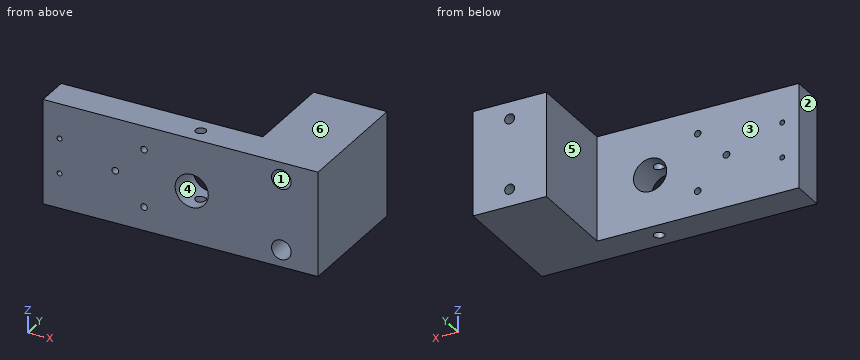
from build123d import *

# Parameters (mm, degrees)
SKETCH2_W                = 40
SKETCH2_H                = 12.7
BOSS_EXTRUDE1_DEPTH      = 105.35
SKETCH4_R                = 6.35
CUT_EXTRUDE1_DEPTH       = 13.7
F_4_0_4_DIAMETER_HOLE1_D = 4
SKETCH9_R                = 1.291519898
SKETCH9_R_2              = 1.25
CUT_EXTRUDE3_DEPTH       = 13.7000001
SKETCH14_W               = 28.1
SKETCH14_H               = 40
BOSS_EXTRUDE3_DEPTH      = 35.45
SKETCH10_R               = 3.75
CUT_EXTRUDE4_DEPTH       = 24.5
SKETCH15_R               = 1.905
CUT_EXTRUDE7_DEPTH       = 24.65
SKETCH17_R               = 0.95
CUT_EXTRUDE8_DEPTH       = 21


with BuildPart() as part:
    # Sketch2 → Boss-Extrude1 (new body)
    with BuildSketch(Plane(origin=(0, 0, 0), x_dir=(0, 0, -1), z_dir=(1, 0, 0))):
        with Locations((-8.031139822, -4.466363736)):
            Rectangle(SKETCH2_W, SKETCH2_H)
    extrude(amount=BOSS_EXTRUDE1_DEPTH)

    # Sketch4 → Cut-Extrude1 (cut, through all)
    with BuildSketch(Plane(origin=(0, 1.883636264, 0), x_dir=(1, 0, 0), z_dir=(0, 1, 0))):
        with Locations((56.96, -8.031139822)):
            Circle(SKETCH4_R)
    extrude(amount=-CUT_EXTRUDE1_DEPTH, mode=Mode.SUBTRACT)

    # Ø4.0 (4) Diameter Hole1 (through all)
    with Locations(Plane.XY.offset(28.031139822)):
        with Locations((56.96, -4.466363736)):
            Hole(F_4_0_4_DIAMETER_HOLE1_D / 2)

    # Sketch9 → Cut-Extrude3 (cut, through all)
    with BuildSketch(Plane(origin=(0, 1.883636264, 0), x_dir=(1, 0, 0), z_dir=(0, 1, 0))):
        with Locations((27.7, -8.031139822)):
            Circle(SKETCH9_R)
        with Locations((38.7, 2.968860178)):
            Circle(SKETCH9_R_2)
        with Locations((38.7, -19.031139822)):
            Circle(SKETCH9_R_2)
    extrude(amount=-CUT_EXTRUDE3_DEPTH, mode=Mode.SUBTRACT)

    # Sketch14 → Boss-Extrude3 (add)
    with BuildSketch(Plane(origin=(0, 1.883636264, 0), x_dir=(1, 0, 0), z_dir=(0, 1, 0))):
        with Locations((91.3, -8.031139822)):
            Rectangle(SKETCH14_W, SKETCH14_H)
    extrude(amount=BOSS_EXTRUDE3_DEPTH)

    # Sketch10 → Cut-Extrude4 (cut)
    with BuildSketch(Plane(origin=(0, -10.816363736, 0), x_dir=(1, 0, 0), z_dir=(0, 1, 0))):
        with Locations((91.3, -21.505839822)):
            Circle(SKETCH10_R)
        with Locations((91.3, 5.443560178)):
            Circle(SKETCH10_R)
    extrude(amount=CUT_EXTRUDE4_DEPTH, mode=Mode.SUBTRACT)

    # Sketch15 → Cut-Extrude7 (cut, through all)
    with BuildSketch(Plane.XZ.offset(-13.683636264)):
        with Locations((91.3, -5.443560178)):
            Circle(SKETCH15_R)
        with Locations((91.3, 21.505839822)):
            Circle(SKETCH15_R)
    extrude(amount=-CUT_EXTRUDE7_DEPTH, mode=Mode.SUBTRACT)

    # Sketch17 → Cut-Extrude8 (cut)
    with BuildSketch(Plane.XZ.offset(10.816363736)):
        with Locations((6.35, 14.698139822)):
            Circle(SKETCH17_R)
        with Locations((6.35, 1.364139822)):
            Circle(SKETCH17_R)
    extrude(amount=-CUT_EXTRUDE8_DEPTH, mode=Mode.SUBTRACT)


solid = part.part
Work out the finished part from the listing and answer in its coordinate system (mm). Face numbers are marked on the shaded views. A direction names the side the tool comes from. Coordinates: 2 decimals unless noted, no trailing zeros. Loops run counter-clockwise (first coordinate to the right, second up) from the corner with the lowest first, then second, coordinate; pieces in that order, holes last. Notation, with made-up numbers: M 65.25,50 L 89.25,50 A21 cw 89.25,65 Z; hole C 69,86.5 d9. An arc over 180 degrees is marked long. Answer in a Markdown table with one row per item. Add a question column.
1. The mould has two halves that part along X. Classify the marked faces 4, 5 and 6: pulls with the +X half, pulls with the -X half, needs draft (parallel to the pull), parting line crosses it, or undercut.
2. Find section B-B, the plane x = 27.7. Write down the section's boundary in (y, z).
3. Consider L1, parallel to Z at x = 38.7, y = -6.75; L2, parallel to Z at x = 56.96, y = -1; L3, parallel to Z at x = 90, y = -4. Determine where each line is inside the solid, lowest interval first.
4. Find section A-A, the plane x = 91.3. Write down the section's boundary in (y, z).
5. Flat-ended cylindrical pins translate along their axes: P1, Ø2, axis at y = 17, z = 0.5, coming from the -X side; P2, Ø8, axis at x = 89.5, z = -5, coming from the -Y side; P3, Ø4, axis at x = 38.7, z = 19.03, coming from the +Y side. Find the tip coordinate at first contact, or state that the pin passes through.
6. Find section C-C, the plane x = 56.96. Write down the section's boundary in (y, z), then the cut area to 3 significant figures.
7. A tool of negligible diameter and unlimited length cuts with its end or side. For the marked faces 1, 2 and 3, from which of +Z, -Z, +X, -X, +Y, -Y can it reach the whole face along a straight path? Write none if from no direction.
8. Find section D-D, the plane z = 3.5. Write down the section's boundary in (x, y), then the cut area to 3 significant figures.
Reported:
| question | item | result |
|---|---|---|
| 1 | face 4 | undercut |
| 1 | face 5 | pulls with the -X half |
| 1 | face 6 | needs draft |
| 2 | outline | M -10.82,-11.97 L 1.88,-11.97 L 1.88,6.74 L -10.82,6.74 Z; M -10.82,9.32 L 1.88,9.32 L 1.88,28.03 L -10.82,28.03 Z |
| 3 | L1 | z = -11.97 to -4.22, -1.72 to 17.78, 20.28 to 28.03 |
| 3 | L2 | z = -11.97 to 1.68, 14.38 to 28.03 |
| 3 | L3 | z = -11.97 to -8.96, -1.93 to 17.99, 25.02 to 28.03 |
| 4 | outline | M -10.82,-11.97 L 37.33,-11.97 L 37.33,-7.35 L 13.68,-7.35 L 13.68,-9.19 L -10.82,-9.19 Z; M -10.82,-1.69 L 13.68,-1.69 L 13.68,-3.54 L 37.33,-3.54 L 37.33,19.6 L 13.68,19.6 L 13.68,17.76 L -10.82,17.76 Z; M -10.82,25.26 L 13.68,25.26 L 13.68,23.41 L 37.33,23.41 L 37.33,28.03 L -10.82,28.03 Z |
| 5 | P1 | stops at x = 77.25 |
| 5 | P2 | stops at y = -10.82 |
| 5 | P3 | stops at y = 1.88 |
| 6 | outline | M -10.82,-11.97 L -6.47,-11.97 L -6.47,1.68 L -10.82,1.68 Z; M -10.82,14.38 L -6.47,14.38 L -6.47,28.03 L -10.82,28.03 Z; M -2.47,-11.97 L 1.88,-11.97 L 1.88,1.68 L -2.47,1.68 Z; M -2.47,14.38 L 1.88,14.38 L 1.88,28.03 L -2.47,28.03 Z |
| 6 | area | 238 mm^2 |
| 7 | face 1 | -Y |
| 7 | face 2 | +Z, -Z, -X, +Y, -Y |
| 7 | face 3 | +Z, -Z, -X, +Y |
| 8 | outline | M 0,-10.82 L 52.51,-10.82 L 52.51,1.88 L 0,1.88 Z; M 61.41,-10.82 L 105.35,-10.82 L 105.35,37.33 L 77.25,37.33 L 77.25,1.88 L 61.41,1.88 Z |
| 8 | area | 2,220 mm^2 |
